Check sheet for the modelled part. Datum: model origin and axes. Units: mm. Coordinates: 2 decimals unless noted, no trailing zeros. Loops run counter-clockwise (first coordinate to the right, second up) from the corner with the lowest first, then second, coordinate; pieces in that order, holes last. Notation, with made-up numbers: (-14.75, 52) -> (37.25, 52) arc R20 ccw to (37.25, 80) -> close; hole circle Ø11 at (-12, 4.25). An arc over 180 degrees is marked (long way). Use one line per item in the form item = value.
from build123d import *

# Parameters (mm, degrees)
BOSS_EXTRUDE1_DEPTH     = 4
FILLET1_R               = 0.5
CHAMFER1_SIZE           = 0.5
SKETCH2_R               = 4
CUT_EXTRUDE1_DEPTH      = 4
CUT_EXTRUDE1_DEPTH_BACK = 4


with BuildPart() as part:
    # Sketch1 → Boss-Extrude1 (new body)
    with BuildSketch(Plane(origin=(0, 0, 0), x_dir=(1, 0, 0), z_dir=(0, 1, 0))):
        Polygon((6.003079224, 5.412612415), (-1.68592024, 7.905125317), (-7.688999465, 2.492512902), (-6.003079224, -5.412612415), (1.68592024, -7.905125317), (7.688999465, -2.492512902), align=None)
    extrude(amount=BOSS_EXTRUDE1_DEPTH)

    # Fillet1
    fillet1_edges = [part.edges().sort_by_distance(p)[0] for p in [
        (7.688999465, 2, 2.492512902),
        (1.68592024, 2, 7.905125317),
        (-6.003079224, 2, 5.412612415),
        (-7.688999465, 2, -2.492512902),
        (-1.68592024, 2, -7.905125317),
        (6.003079224, 2, -5.412612415),
    ]]
    fillet(fillet1_edges, radius=FILLET1_R)

    # Chamfer1
    chamfer1_edges = [part.edges().sort_by_distance(p)[0] for p in [
        (6.846039345, 4, -1.460049757),
        (4.687459853, 4, 5.198819109),
        (2.158579492, 4, -6.658868866),
        (-4.687459853, 4, -5.198819109),
        (-6.846039345, 4, 1.460049757),
        (-2.158579492, 4, 6.658868866),
        (1.669786634, 4, 7.829476319),
        (5.945632073, 4, -5.360815804),
        (-1.669786634, 4, -7.829476319),
        (-7.615418708, 4, -2.468660515),
        (-5.945632073, 4, 5.360815804),
        (7.615418708, 4, 2.468660515),
    ]]
    chamfer(chamfer1_edges, length=CHAMFER1_SIZE)

    # Sketch2 → Cut-Extrude1 (cut, two sides)
    with BuildSketch(Plane(origin=(0, 4, 0), x_dir=(1, 0, 0), z_dir=(0, 1, 0))) as cut_extrude1_sk:
        Circle(SKETCH2_R)
    extrude(amount=CUT_EXTRUDE1_DEPTH, mode=Mode.SUBTRACT)
    extrude(cut_extrude1_sk.sketch, amount=-CUT_EXTRUDE1_DEPTH_BACK, mode=Mode.SUBTRACT)


solid = part.part
(1) Section check B-B, the plane z = 0. Record the boundary of the cut face in (x, y), plus the area to 3 significant figures.
Established:
outline = (-7.16, 0) -> (-4, 0) -> (-4, 4) -> (-6.65, 4) -> (-7.16, 3.5) -> close; (4, 0) -> (7.16, 0) -> (7.16, 3.5) -> (6.65, 4) -> (4, 4) -> close
area = 25.0 mm²
(2) Section check D-D, the plane y = 3.7. Record the boundary of the cut face in (x, z).
Established:
outline = (-7.43, -2.25) arc R0.3 ccw to (-7.34, -2.54) -> (-1.77, -7.56) arc R0.3 ccw to (-1.47, -7.63) -> (5.67, -5.31) arc R0.3 ccw to (5.87, -5.09) -> (7.43, 2.25) arc R0.3 ccw to (7.34, 2.54) -> (1.77, 7.56) arc R0.3 ccw to (1.47, 7.63) -> (-5.67, 5.31) arc R0.3 ccw to (-5.87, 5.09) -> close; hole circle Ø8 at (0, 0)
(3) Scan lines: line 1 along Z through (x, y) = (2.5, 0.55); line 2 along X through (y, z) = (2, 0); line 3 along X through (y, z) = (2.85, 1.5). Record each from-to range of solid material in increasing order.
Established:
line_1 = -6.55 to -3.12, 3.12 to 7.17
line_2 = -7.16 to -4, 4 to 7.16
line_3 = -6.84 to -3.71, 3.71 to 7.48
(4) Go/stop test with flat-tipped pins: P1, Ø1, axis at x = -1, y = 2.5, coming from the +Z side; P2, Ø5, axis at x = -0.5, z = 4, coming from the -Y side. Record where each tip stops, or that it passes through.
Established:
P1 = 7.2
P2 = 0
(5) Mould release check, pull along Z, two halves, no side actions. Record for faces 1 (the flat face through (-4.5, 3.7, -5.1)), 2 (the flat face through (-2.209, 1.726, 6.643)), 3 (the cylindrical face through (-0.867, 2.028, 3.905)): +Z half, -Z half, draft (parallel to the pull), parting line (faces both ways), or undercut.
Established:
face_1 = -Z half
face_2 = +Z half
face_3 = undercut
(6) Section check A-A, the plane y = 0.75. Record the boundary of the cut face in (x, z), plus the area to 3 significant figures.
Established:
outline = (-7.63, -2.21) arc R0.5 ccw to (-7.47, -2.69) -> (-1.9, -7.71) arc R0.5 ccw to (-1.41, -7.82) -> (5.73, -5.5) arc R0.5 ccw to (6.06, -5.13) -> (7.63, 2.21) arc R0.5 ccw to (7.47, 2.69) -> (1.9, 7.71) arc R0.5 ccw to (1.41, 7.82) -> (-5.73, 5.5) arc R0.5 ccw to (-6.06, 5.13) -> close; hole circle Ø8 at (0, 0)
area = 119 mm²
(7) Section check C-C, the plane x = -2.5. Record the boundary of the cut face in (y, z).
Established:
outline = (0, -7.17) -> (3.5, -7.17) -> (4, -6.5) -> (4, -3.12) -> (0, -3.12) -> close; (0, 3.12) -> (4, 3.12) -> (4, 6.02) -> (3.5, 6.55) -> (0, 6.55) -> close
